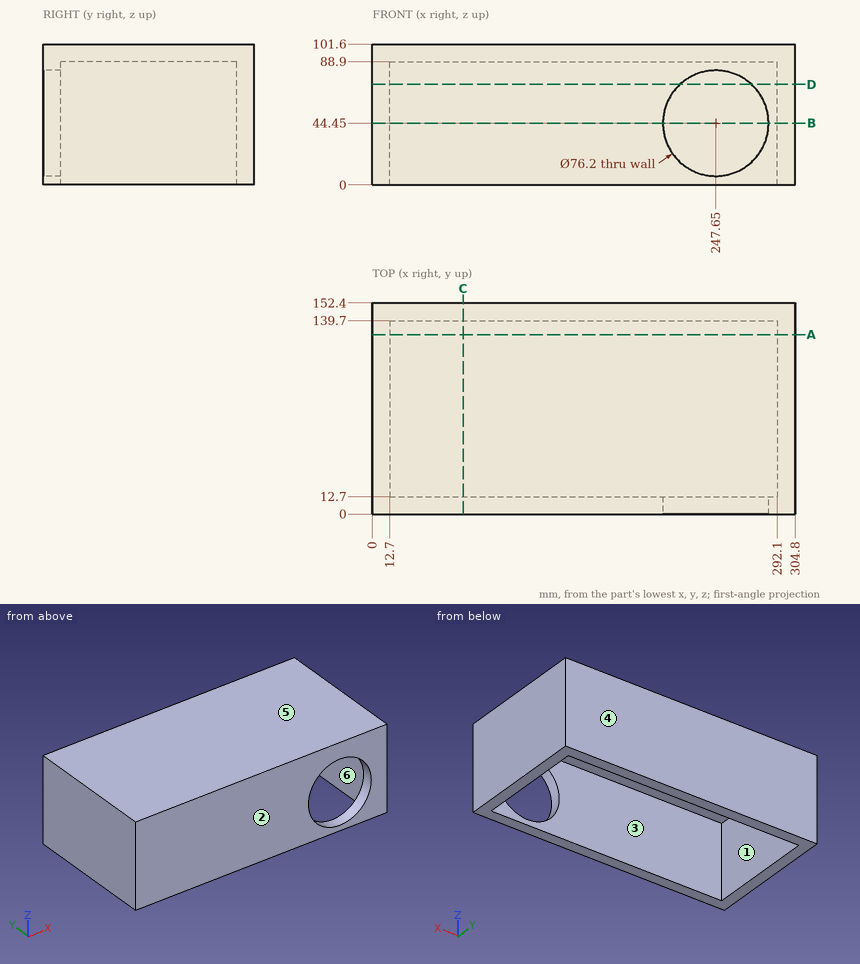
Can you work these out from the drawing? Everything is in mm from the part's minimum corner. A direction names the side the tool comes from. Coordinates: 2 decimals unless noted, no trailing zeros. Write each loop counter-clockwise with the first axis right and the second up, starting at its lowest first coordinate (ties: lowest second). Pieces come first, ordered by that corner, then holes. Notation, with made-up numbers: (2.25, -9.75) -> (28.25, -9.75) arc R25 ccw to (28.25, 18.25) -> close; hole circle Ø2 at (1, 52.5). An arc over 180 degrees is marked (long way). Return JSON: item names as keys, results as strings.
(1) Which directions (+Z, -Z, +X, -X, +Y, -Y) give clear straight access to the entire face, cutting with the end or side of a thin tool? Please do the marked faces 1 and 2.
Numbers:
{"face 1": "-Z", "face 2": "+Z, -Z, +X, -X, -Y"}
(2) Imagine slicing it at A-A, the plane y = 129.5. Please give me the cut outline in (x, z), then the cut area to 3 significant figures.
Numbers:
{"outline": "(0, 0) -> (12.7, 0) -> (12.7, 88.9) -> (292.1, 88.9) -> (292.1, 0) -> (304.8, 0) -> (304.8, 101.6) -> (0, 101.6) -> close", "area": "6,130 mm2"}
(3) Imagine slicing it at B-B, the plane z = 44.45. Please give me the cut outline in (x, y).
Numbers:
{"outline": "(0, 0) -> (209.55, 0) -> (209.55, 12.7) -> (12.7, 12.7) -> (12.7, 139.7) -> (292.1, 139.7) -> (292.1, 12.7) -> (285.75, 12.7) -> (285.75, 0) -> (304.8, 0) -> (304.8, 152.4) -> (0, 152.4) -> close"}
(4) Imagine slicing it at D-D, the plane z = 72.5. Please give me the cut outline in (x, y).
Numbers:
{"outline": "(0, 0) -> (221.87, 0) -> (221.87, 12.7) -> (12.7, 12.7) -> (12.7, 139.7) -> (292.1, 139.7) -> (292.1, 12.7) -> (273.43, 12.7) -> (273.43, 0) -> (304.8, 0) -> (304.8, 152.4) -> (0, 152.4) -> close"}
(5) I'm going to push flat-ended pins straight in: pin 1 (2 mm diameter, centred on x = 103, z = 91, fed in from -Y); pin 2 (2 mm diameter, centred on x = 209.5, y = 67, fed in from -Z); pin 3 (4 mm diameter, centred on x = 229.5, z = 51, fed in from -Y). Where does each tip first touch, or does it pass through?
Numbers:
{"pin 1": "stops at y = 0", "pin 2": "stops at z = 88.9", "pin 3": "stops at y = 139.7"}
(6) We'd pull the mould along Y, two halves only. Please class the marked faces 3, 4, 5 and 6: +Y half, -Y half, draft (parallel to the pull), parting line (faces both ways), or undercut.
Numbers:
{"face 3": "undercut", "face 4": "+Y half", "face 5": "draft", "face 6": "undercut"}
(7) I need wall thicknesses on L1, parallel to X at y = 24, z = 84.5; L2, parallel to Y at x = 103.5, z = 55; L3, parallel to X at y = 3, z = 44. Which ranges of each line are inside material? Lowest first, please.
Numbers:
{"L1": "x = 0 to 12.7, 292.1 to 304.8", "L2": "y = 0 to 12.7, 139.7 to 152.4", "L3": "x = 0 to 209.55, 285.75 to 304.8"}
(8) Imagine slicing it at C-C, the plane x = 65.5. Please give me the cut outline in (y, z), then the cut area to 3 significant figures.
Numbers:
{"outline": "(0, 0) -> (12.7, 0) -> (12.7, 88.9) -> (139.7, 88.9) -> (139.7, 0) -> (152.4, 0) -> (152.4, 101.6) -> (0, 101.6) -> close", "area": "4,190 mm2"}
